Here's how the part is built. I have some questions about the finished solid (model axes, mm). Face numbers are marked on the shaded views. A direction names the side the tool comes from. Round coordinates to 2 decimals unless told otherwise and drop trailing zeros. Write each loop counter-clockwise with the first axis right and the second up, starting at its lowest first coordinate (ties: lowest second). Pieces come first, ordered by that corner, then holes. Notation, with made-up numbers: (39, 49) -> (56, 49) arc R26 cw to (56, 87) -> close; hole circle Ø11 at (84.25, 75.5). An arc over 180 degrees is marked (long way). Answer in a Markdown table with one row per item.
from build123d import *

# Parameters (mm, degrees)
SKETCH3_R             = 2.85
BOSS_EXTRUDE3_DEPTH   = 1.5
BOSS_EXTRUDE3_2_DEPTH = 1.5
SKETCH2_W             = 121.8
SKETCH2_H             = 30
BOSS_EXTRUDE2_DEPTH   = 1.2
FILLET1_R             = 5


with BuildPart() as part:
    # Sketch3 → Boss-Extrude3 (new body)
    with BuildSketch(Plane.XY):
        with BuildLine():
            Line((-7.997540574, -43.228135601), (-8, -43.4))
            Line((-8, -43.4), (-8, -53.4))
            ThreePointArc((-8, -53.4), (-7.121320344, -55.521320344), (-5, -56.4))
            Line((-5, -56.4), (5, -56.4))
            ThreePointArc((5, -56.4), (7.121320344, -55.521320344), (8, -53.4))
            Line((8, -53.4), (8, -43.4))
            Line((8, -43.4), (7.997540574, -43.228135601))
            ThreePointArc((7.997540574, -43.228135601), (7.060914023, -41.218251724), (5, -40.4))
            Line((5, -40.4), (-5, -40.4))
            ThreePointArc((-5, -40.4), (-7.060914023, -41.218251724), (-7.997540574, -43.228135601))
        make_face()
        with Locations((0, -47.952381154)):
            Circle(SKETCH3_R, mode=Mode.SUBTRACT)
    extrude(amount=BOSS_EXTRUDE3_DEPTH)



with BuildPart() as body_2:
    # Sketch3 → Boss-Extrude3 2 (new body)
    with BuildSketch(Plane.XY):
        with BuildLine():
            Line((110.8, -40.4), (100.8, -40.4))
            ThreePointArc((100.8, -40.4), (98.739085977, -41.218251724), (97.802459426, -43.228135601))
            Line((97.802459426, -43.228135601), (97.8, -43.4))
            Line((97.8, -43.4), (97.8, -53.4))
            ThreePointArc((97.8, -53.4), (98.678679656, -55.521320344), (100.8, -56.4))
            Line((100.8, -56.4), (110.8, -56.4))
            ThreePointArc((110.8, -56.4), (112.921320344, -55.521320344), (113.8, -53.4))
            Line((113.8, -53.4), (113.8, -43.4))
            Line((113.8, -43.4), (113.797540574, -43.228135601))
            ThreePointArc((113.797540574, -43.228135601), (112.860914023, -41.218251724), (110.8, -40.4))
        make_face()
        with Locations((105.8, -47.952381154)):
            Circle(SKETCH3_R, mode=Mode.SUBTRACT)
    extrude(amount=BOSS_EXTRUDE3_2_DEPTH)


with BuildPart() as part_1:
    add(part.part)

    add(body_2.part)  # Boss-Extrude2 merges body 2
    # Sketch2 → Boss-Extrude2 (add)
    with BuildSketch(Plane.XZ.offset(56.4)):
        with Locations((52.9, 14)):
            Rectangle(SKETCH2_W, SKETCH2_H)
    extrude(amount=BOSS_EXTRUDE2_DEPTH)

    # Fillet1
    fillet1_edges = [part_1.edges().sort_by_distance(p)[0] for p in [
        (-8, -57, 29),
        (-8, -57, -1),
        (113.8, -57, -1),
        (113.8, -57, 29),
    ]]
    fillet(fillet1_edges, radius=FILLET1_R)


solid = part_1.part
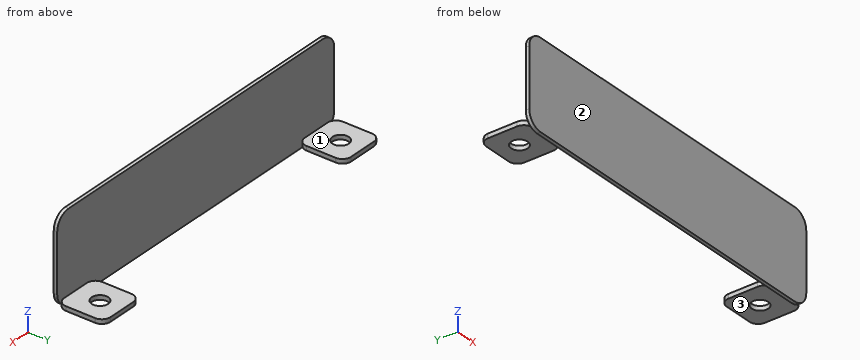
1) I want a section at A-A, the plane x = 105.8. List the corners of the cut face in (y, z) for me, and give its area (4 significant figures).
Response:
| item | result |
|---|---|
| outline | (-57.6, -1) -> (-56.4, -1) -> (-56.4, 0) -> (-50.8, 0) -> (-50.8, 1.5) -> (-56.4, 1.5) -> (-56.4, 29) -> (-57.6, 29) -> close; (-45.1, 0) -> (-40.4, 0) -> (-40.4, 1.5) -> (-45.1, 1.5) -> close |
| area | 51.45 mm^2 |
2) I want a section at C-C, the plane x = 62. List the corners of the cut face in (y, z) for me.
Response:
| item | result |
|---|---|
| outline | (-57.6, -1) -> (-56.4, -1) -> (-56.4, 29) -> (-57.6, 29) -> close |
3) I want a section at B-B, the plane z = 9. List the corners of the cut face in (x, y) for me.
Response:
| item | result |
|---|---|
| outline | (-8, -57.6) -> (113.8, -57.6) -> (113.8, -56.4) -> (-8, -56.4) -> close |
4) For pin 1 (5 mm diameter, centred on x = 106, y = -44.5, fed in from +Z); pin 2 (8 mm diameter, centred on x = 109, y = -48.5, fed in from -Z); pin 3 (3.5 mm diameter, centred on x = 0, y = -47.95, fed in from -Z); pin 4 (15 mm diameter, centred on x = 62, z = 13.5, fed in from +Y), each with a flat end and sliding along its axis, tell me the tip position at first contact or that it passes through.
Response:
| item | result |
|---|---|
| pin 1 | stops at z = 1.5 |
| pin 2 | stops at z = 0 |
| pin 3 | passes through |
| pin 4 | stops at y = -56.4 |
5) I need wall thicknesses on line 1 (Y direction, x = 0, z = 0.55); line 2 (X direction, y = -52.25, z = 1); line 3 (Y direction, x = 40, z = 19.25). Which ranges of each line are inside material? Lowest first, please. Write a range as [from, to].
Response:
| item | result |
|---|---|
| line 1 | y = [-57.6, -50.8], [-45.1, -40.4] |
| line 2 | x = [-8, 8], [97.8, 113.8] |
| line 3 | y = [-57.6, -56.4] |
6) Which directions (+Z, -Z, +X, -X, +Y, -Y) give clear straight access to the entire face, cutting with the end or side of a thin tool? Please do the marked faces 1, 2 and 3.
Response:
| item | result |
|---|---|
| face 1 | +Z, +X, -X, +Y |
| face 2 | +Z, -Z, +X, -X, -Y |
| face 3 | -Z, +X, -X, +Y |
